Geometry check sheet. Reference: the model listing, model coordinates, mm. A direction names the side the tool comes from. Round coordinates to 2 decimals unless told otherwise and drop trailing zeros. Write each loop counter-clockwise with the first axis right and the second up, starting at its lowest first coordinate (ties: lowest second). Pieces come first, ordered by that corner, then holes. Notation, with made-up numbers: M 29,22.5 L 57,22.5 A25 cw 57,47.5 Z; hole C 26.5,37 d1. An arc over 180 degrees is marked long. Answer in a Markdown table with one row per item. Add a question column.
from build123d import *

# Parameters (mm, degrees)
EXTRUDE1_DEPTH             = 125
EXTRUDE2_DEPTH             = 5.5
EXTRUDE3_DEPTH             = 5.5
SKETCH4_R                  = 32.5
EXTRUDE5_DEPTH             = 101
EXTRUDE7_DEPTH             = 80
SKETCH7_R                  = 2.5
EXTRUDE9_DEPTH             = 15
LPATTERN1_COUNT            = 2
LPATTERN1_PITCH            = 56
LPATTERN2_COUNT            = 2
LPATTERN2_PITCH            = 56
LPATTERN2_COPY_1_SKETCH_R  = 2.5
LPATTERN2_COPY_1_DEPTH     = 15
EXTRUDE10_DEPTH            = 1
EXTRUDE11_DEPTH            = 3
SKETCH10_R                 = 23.5
EXTRUDE12_DEPTH            = 24
SKETCH11_R                 = 21
EXTRUDE13_DEPTH            = 84
SKETCH12_R                 = 23.5
EXTRUDE14_DEPTH            = 24
SKETCH13_R                 = 2.5
EXTRUDE15_DEPTH            = 20
LPATTERN3_COUNT            = 2
LPATTERN3_PITCH            = 43
LPATTERN4_COUNT            = 2
LPATTERN4_PITCH            = 43
LPATTERN4_COPY_1_SKETCH_R  = 2.5
LPATTERN4_COPY_1_DEPTH     = 20
SKETCH14_R                 = 2.5
EXTRUDE16_DEPTH            = 20
LPATTERN5_COUNT            = 2
LPATTERN5_PITCH            = 76
LPATTERN6_COUNT            = 2
LPATTERN6_PITCH            = 76
LPATTERN6_COPY_1_SKETCH_R  = 2.5
LPATTERN6_COPY_1_DEPTH     = 20
SKETCH15_R                 = 2.5
EXTRUDE17_DEPTH            = 20
LPATTERN7_COUNT            = 2
LPATTERN7_PITCH            = 76
LPATTERN8_COUNT            = 2
LPATTERN8_PITCH            = 76
LPATTERN8_COPY_1_SKETCH_R  = 2.5
LPATTERN8_COPY_1_DEPTH     = 20
SKETCH18_R                 = 2.5
EXTRUDE20_DEPTH            = 20
LPATTERN9_COUNT            = 2
LPATTERN9_PITCH            = 56
LPATTERN10_COUNT           = 2
LPATTERN10_PITCH           = 56
LPATTERN10_COPY_1_SKETCH_R = 2.5
LPATTERN10_COPY_1_DEPTH    = 20


with BuildPart() as part:
    # Sketch1 → Extrude1 (new body)
    with BuildSketch(Plane(origin=(0, 0, 0), x_dir=(1, 0, 0), z_dir=(0, 1, 0))):
        Polygon((0, 0), (0, 81), (4, 85), (99, 85), (103, 81), (103, 0), (99, -4), (4, -4), align=None)
    extrude(amount=EXTRUDE1_DEPTH)

    # Sketch2 → Extrude2 (add)
    with BuildSketch(Plane.XY.offset(4)):
        Polygon((22, 82), (81, 82), (90, 73), (90, 14), (81, 5), (22, 5), (13, 14), (13, 73), align=None)
    extrude(amount=EXTRUDE2_DEPTH)

    # Sketch3 → Extrude3 (add)
    with BuildSketch(Plane(origin=(0, 0, -85), x_dir=(-1, 0, 0), z_dir=(0, 0, -1))):
        Polygon((-81, 82), (-22, 82), (-13, 73), (-13, 14), (-22, 5), (-81, 5), (-90, 14), (-90, 73), align=None)
    extrude(amount=EXTRUDE3_DEPTH)

    # Sketch4 → Extrude5 (cut, through all)
    with BuildSketch(Plane.XY.offset(9.5)):
        with Locations((51.5, 43.5)):
            Circle(SKETCH4_R)
    extrude(amount=-EXTRUDE5_DEPTH, mode=Mode.SUBTRACT)

    # Sketch5 → Extrude7 (cut)
    with BuildSketch(Plane.XY.offset(-0.5)):
        Polygon((10, 10), (93, 10), (93, 65), (79, 65), (79, 110), (24, 110), (24, 65), (10, 65), align=None)
    extrude(amount=-EXTRUDE7_DEPTH, mode=Mode.SUBTRACT)

    # Sketch7 → Extrude9 (cut)
    with BuildSketch(Plane.XY.offset(9.5)):
        with Locations((23.5, 71.5)):
            Circle(SKETCH7_R)
    extrude9 = extrude(amount=-EXTRUDE9_DEPTH, mode=Mode.SUBTRACT)

    # LPattern1: Extrude9 ×2
    with Locations(*[(i * LPATTERN1_PITCH, 0, 0) for i in range(1, LPATTERN1_COUNT)]):
        add(extrude9, mode=Mode.SUBTRACT)

    # LPattern2: Extrude9 ×2
    with Locations(*[(0, -i * LPATTERN2_PITCH, 0) for i in range(1, LPATTERN2_COUNT)]):
        add(extrude9, mode=Mode.SUBTRACT)

    # LPattern2 copy 1 sketch → LPattern2 copy 1 (cut)
    with BuildSketch(Plane(origin=(56, -56, 9.5), x_dir=(1, 0, 0), z_dir=(0, 0, 1))):
        with Locations((23.5, 71.5)):
            Circle(LPATTERN2_COPY_1_SKETCH_R)
    extrude(amount=-LPATTERN2_COPY_1_DEPTH, mode=Mode.SUBTRACT)

    # Sketch8 → Extrude10 (add)
    with BuildSketch(Plane(origin=(103, 0, 0), x_dir=(0, 0, -1), z_dir=(1, 0, 0))):
        Polygon((6, 115), (75, 115), (81, 109), (81, 46), (75, 40), (6, 40), (0, 46), (0, 109), align=None)
    extrude(amount=EXTRUDE10_DEPTH)

    # Sketch9 → Extrude11 (add)
    with BuildSketch(Plane.ZY):
        Polygon((-75, 115), (-6, 115), (0, 109), (0, 46), (-6, 40), (-75, 40), (-81, 46), (-81, 109), align=None)
    extrude(amount=EXTRUDE11_DEPTH)

    # Sketch10 → Extrude12 (cut)
    with BuildSketch(Plane(origin=(104, 0, 0), x_dir=(0, 0, -1), z_dir=(1, 0, 0))):
        with Locations((40.5, 77.5)):
            Circle(SKETCH10_R)
    extrude(amount=-EXTRUDE12_DEPTH, mode=Mode.SUBTRACT)

    # Sketch11 → Extrude13 (cut, through all)
    with BuildSketch(Plane(origin=(80, 0, 0), x_dir=(0, 0, -1), z_dir=(1, 0, 0))):
        with Locations((40.5, 77.5)):
            Circle(SKETCH11_R)
    extrude(amount=-EXTRUDE13_DEPTH, mode=Mode.SUBTRACT)

    # Sketch12 → Extrude14 (cut)
    with BuildSketch(Plane.ZY.offset(3)):
        with Locations((-40.5, 77.5)):
            Circle(SKETCH12_R)
    extrude(amount=-EXTRUDE14_DEPTH, mode=Mode.SUBTRACT)

    # Sketch13 → Extrude15 (cut)
    with BuildSketch(Plane(origin=(104, 0, 0), x_dir=(0, 0, -1), z_dir=(1, 0, 0))):
        with Locations((19, 99)):
            Circle(SKETCH13_R)
    extrude15 = extrude(amount=-EXTRUDE15_DEPTH, mode=Mode.SUBTRACT)

    # LPattern3: Extrude15 ×2
    with Locations(*[(0, 0, -i * LPATTERN3_PITCH) for i in range(1, LPATTERN3_COUNT)]):
        add(extrude15, mode=Mode.SUBTRACT)

    # LPattern4: Extrude15 ×2
    with Locations(*[(0, -i * LPATTERN4_PITCH, 0) for i in range(1, LPATTERN4_COUNT)]):
        add(extrude15, mode=Mode.SUBTRACT)

    # LPattern4 copy 1 sketch → LPattern4 copy 1 (cut)
    with BuildSketch(Plane(origin=(104, -43, -43), x_dir=(0, 0, -1), z_dir=(1, 0, 0))):
        with Locations((19, 99)):
            Circle(LPATTERN4_COPY_1_SKETCH_R)
    extrude(amount=-LPATTERN4_COPY_1_DEPTH, mode=Mode.SUBTRACT)

    # Sketch14 → Extrude16 (cut)
    with BuildSketch(Plane(origin=(0, 125, 0), x_dir=(1, 0, 0), z_dir=(0, 1, 0))):
        with Locations((13.5, 78.5)):
            Circle(SKETCH14_R)
    extrude16 = extrude(amount=-EXTRUDE16_DEPTH, mode=Mode.SUBTRACT)

    # LPattern5: Extrude16 ×2
    with Locations(*[(i * LPATTERN5_PITCH, 0, 0) for i in range(1, LPATTERN5_COUNT)]):
        add(extrude16, mode=Mode.SUBTRACT)

    # LPattern6: Extrude16 ×2
    with Locations(*[(0, 0, i * LPATTERN6_PITCH) for i in range(1, LPATTERN6_COUNT)]):
        add(extrude16, mode=Mode.SUBTRACT)

    # LPattern6 copy 1 sketch → LPattern6 copy 1 (cut)
    with BuildSketch(Plane(origin=(76, 125, 76), x_dir=(1, 0, 0), z_dir=(0, 1, 0))):
        with Locations((13.5, 78.5)):
            Circle(LPATTERN6_COPY_1_SKETCH_R)
    extrude(amount=-LPATTERN6_COPY_1_DEPTH, mode=Mode.SUBTRACT)

    # Sketch15 → Extrude17 (cut)
    with BuildSketch(Plane.XZ):
        with Locations((13.5, -2.5)):
            Circle(SKETCH15_R)
    extrude17 = extrude(amount=-EXTRUDE17_DEPTH, mode=Mode.SUBTRACT)

    # LPattern7: Extrude17 ×2
    with Locations(*[(i * LPATTERN7_PITCH, 0, 0) for i in range(1, LPATTERN7_COUNT)]):
        add(extrude17, mode=Mode.SUBTRACT)

    # LPattern8: Extrude17 ×2
    with Locations(*[(0, 0, -i * LPATTERN8_PITCH) for i in range(1, LPATTERN8_COUNT)]):
        add(extrude17, mode=Mode.SUBTRACT)

    # LPattern8 copy 1 sketch → LPattern8 copy 1 (cut)
    with BuildSketch(Plane(origin=(76, 0, -76), x_dir=(1, 0, 0), z_dir=(0, -1, 0))):
        with Locations((13.5, -2.5)):
            Circle(LPATTERN8_COPY_1_SKETCH_R)
    extrude(amount=-LPATTERN8_COPY_1_DEPTH, mode=Mode.SUBTRACT)

    # Sketch18 → Extrude20 (cut)
    with BuildSketch(Plane(origin=(0, 0, -90.5), x_dir=(-1, 0, 0), z_dir=(0, 0, -1))):
        with Locations((-79.5, 71.5)):
            Circle(SKETCH18_R)
    extrude20 = extrude(amount=-EXTRUDE20_DEPTH, mode=Mode.SUBTRACT)

    # LPattern9: Extrude20 ×2
    with Locations(*[(-i * LPATTERN9_PITCH, 0, 0) for i in range(1, LPATTERN9_COUNT)]):
        add(extrude20, mode=Mode.SUBTRACT)

    # LPattern10: Extrude20 ×2
    with Locations(*[(0, -i * LPATTERN10_PITCH, 0) for i in range(1, LPATTERN10_COUNT)]):
        add(extrude20, mode=Mode.SUBTRACT)

    # LPattern10 copy 1 sketch → LPattern10 copy 1 (cut)
    with BuildSketch(Plane(origin=(-56, -56, -90.5), x_dir=(-1, 0, 0), z_dir=(0, 0, -1))):
        with Locations((-79.5, 71.5)):
            Circle(LPATTERN10_COPY_1_SKETCH_R)
    extrude(amount=-LPATTERN10_COPY_1_DEPTH, mode=Mode.SUBTRACT)


solid = part.part
Item 1: Access from +Z, -Z, +X, -X, +Y, -Y to the whole of each face (thin tool, end or side, straight path). Record for faces 1 (the flat face through (17, 10, -88)), 2 (the flat face through (-1, 112, -78)), 3 (the flat face through (17, 65, -69)), 4 (the flat face through (86, 77, -88)), 5 (the cylindrical face through (21.115, 72.251, -82.862)).
Item 2: Section check B-B, the plane x = 37. Record the boundary of the cut face in (y, z).
Item 3: Section check D-D, the plane z = -28.5. Record the boundary of the cut face in (x, y), and give its area (3 significant figures).
Item 4: Gauge pin test, flat ends, axial feed: pin 1 Ø0.5 at (x, z) = (103.5, -37.5) entering from +Y; pin 2 Ø1.5 at (x, y) = (-1.5, 64) entering from -Z; pin 3 Ø3 at (x, z) = (65.5, -87) entering from -Y. Record the tip position at first contact, or that the pin passes through.
Item 5: Section check A-A, the plane z = -40.5. Record the boundary of the cut face in (x, y), and give its area (3 significant figures).
Item 6: Mould release check, pull along Z, two halves, no side actions. Record for faces 6 (the cylindrical face through (22.52, 98.49, -41.15)), 7 (the cylindrical face through (81.885, 72.251, 3.772)), 8 (the flat face through (85, 44, -90.5)): +Z half, -Z half, draft (parallel to the pull), parting line (faces both ways), or undercut.
Item 7: Scan lines: probe 1 along Y at (x, z) = (79.5, -11); probe 2 along X at (y, z) = (20, -61); probe 3 along Y at (x, z) = (57.5, -10). Record each from-to range of solid material in increasing order. Write a range as from..to.
Item 8: Section check C-C, the plane x = 58.5. Record the boundary of the cut face in (y, z).
Result sheet:
| question | item | result |
|---|---|---|
| 1 | face 1 | -Z, -X, -Y |
| 1 | face 2 | -Z, -X, +Y |
| 1 | face 3 | none |
| 1 | face 4 | -Z, +X, +Y |
| 1 | face 5 | -Z |
| 2 | outline | M 0,-85 L 5,-85 L 5,-90.5 L 14.41,-90.5 L 14.41,-80.5 L 10,-80.5 L 10,-0.5 L 14.41,-0.5 L 14.41,9.5 L 5,9.5 L 5,4 L 0,4 Z; M 72.59,-90.5 L 82,-90.5 L 82,-85 L 125,-85 L 125,4 L 82,4 L 82,9.5 L 72.59,9.5 L 72.59,-0.5 L 110,-0.5 L 110,-80.5 L 72.59,-80.5 Z |
| 3 | outline | M -3,40 L 0,40 L 0,0 L 103,0 L 103,40 L 104,40 L 104,57.29 L 93,57.29 L 93,10 L 10,10 L 10,57.29 L -3,57.29 Z; M -3,97.71 L 21,97.71 L 21,94.73 L 24,94.73 L 24,110 L 79,110 L 79,94.73 L 80,94.73 L 80,97.71 L 104,97.71 L 104,115 L 103,115 L 103,125 L 0,125 L 0,115 L -3,115 Z |
| 3 | area | 4,260 mm^2 |
| 4 | pin 1 | stops at y = 115 |
| 4 | pin 2 | stops at z = -81 |
| 4 | pin 3 | stops at y = 5 |
| 5 | outline | M -3,40 L 0,40 L 0,0 L 103,0 L 103,40 L 104,40 L 104,54 L 93,54 L 93,10 L 10,10 L 10,54 L -3,54 Z; M -3,101 L 21,101 L 21,98.5 L 24,98.5 L 24,110 L 79,110 L 79,98.5 L 80,98.5 L 80,101 L 104,101 L 104,115 L 103,115 L 103,125 L 0,125 L 0,115 L -3,115 Z |
| 5 | area | 4,010 mm^2 |
| 6 | face 6 | undercut |
| 6 | face 7 | draft |
| 6 | face 8 | -Z half |
| 7 | probe 1 | y = 0..10, 65..125 |
| 7 | probe 2 | x = 0..10, 93..103 |
| 7 | probe 3 | y = 0..10, 110..125 |
| 8 | outline | M 0,-85 L 5,-85 L 5,-90.5 L 11.76,-90.5 L 11.76,-80.5 L 10,-80.5 L 10,-0.5 L 11.76,-0.5 L 11.76,9.5 L 5,9.5 L 5,4 L 0,4 Z; M 75.24,-90.5 L 82,-90.5 L 82,-85 L 125,-85 L 125,4 L 82,4 L 82,9.5 L 75.24,9.5 L 75.24,-0.5 L 110,-0.5 L 110,-80.5 L 75.24,-80.5 Z |
